```python
from build123d import *

# Parameters (mm, degrees)
SKETCH3_W           = 4
SKETCH3_H           = 0.5
BOSS_EXTRUDE1_DEPTH = 52.5
SKETCH4_R           = 0.6
CUT_EXTRUDE1_DEPTH  = 0.5
SKETCH5_R           = 0.6
CUT_EXTRUDE2_DEPTH  = 0.5
SKETCH6_R           = 0.6
CUT_EXTRUDE3_DEPTH  = 0.5
SKETCH7_R           = 0.6
CUT_EXTRUDE4_DEPTH  = 0.5
SKETCH8_R           = 0.6
CUT_EXTRUDE5_DEPTH  = 0.5
SKETCH9_R           = 0.6
CUT_EXTRUDE6_DEPTH  = 0.5
SKETCH10_R          = 0.6
CUT_EXTRUDE7_DEPTH  = 0.5
SKETCH11_R          = 0.6
CUT_EXTRUDE8_DEPTH  = 0.5
SKETCH12_R          = 0.6
CUT_EXTRUDE9_DEPTH  = 0.5
SKETCH13_R          = 0.6
CUT_EXTRUDE10_DEPTH = 0.5
SKETCH14_R          = 0.6
CUT_EXTRUDE11_DEPTH = 0.5
SKETCH15_R          = 0.6
CUT_EXTRUDE12_DEPTH = 0.5
SKETCH16_R          = 0.6
CUT_EXTRUDE13_DEPTH = 0.5
SKETCH17_R          = 0.6
CUT_EXTRUDE14_DEPTH = 0.5
SKETCH18_R          = 0.6
CUT_EXTRUDE15_DEPTH = 0.5
SKETCH19_R          = 0.6
CUT_EXTRUDE16_DEPTH = 0.5
SKETCH20_R          = 0.6
CUT_EXTRUDE17_DEPTH = 0.5
SKETCH21_R          = 0.6
CUT_EXTRUDE18_DEPTH = 0.5
SKETCH22_R          = 0.6
CUT_EXTRUDE19_DEPTH = 0.5
SKETCH23_R          = 0.6
CUT_EXTRUDE20_DEPTH = 0.3


with BuildPart() as part:
    # Sketch3 → Boss-Extrude1 (new body)
    with BuildSketch(Plane(origin=(0, 0, 0), x_dir=(1, 0, 0), z_dir=(0, 1, 0))):
        with Locations((0, 0.1)):
            Rectangle(SKETCH3_W, SKETCH3_H)
    extrude(amount=-BOSS_EXTRUDE1_DEPTH)

    # Sketch4 → Cut-Extrude1 (cut)
    with BuildSketch(Plane.XY.offset(0.15)):
        with Locations((1.25, -3.45)):
            Circle(SKETCH4_R)
    extrude(amount=-CUT_EXTRUDE1_DEPTH, mode=Mode.SUBTRACT)

    # Sketch5 → Cut-Extrude2 (cut)
    with BuildSketch(Plane.XY.offset(0.15)):
        with Locations((1.25, -5.95)):
            Circle(SKETCH5_R)
    extrude(amount=-CUT_EXTRUDE2_DEPTH, mode=Mode.SUBTRACT)

    # Sketch6 → Cut-Extrude3 (cut)
    with BuildSketch(Plane.XY.offset(0.15)):
        with Locations((1.25, -13.6)):
            Circle(SKETCH6_R)
    extrude(amount=-CUT_EXTRUDE3_DEPTH, mode=Mode.SUBTRACT)

    # Sketch7 → Cut-Extrude4 (cut)
    with BuildSketch(Plane.XY.offset(0.15)):
        with Locations((1.25, -16.1)):
            Circle(SKETCH7_R)
    extrude(amount=-CUT_EXTRUDE4_DEPTH, mode=Mode.SUBTRACT)

    # Sketch8 → Cut-Extrude5 (cut)
    with BuildSketch(Plane.XY.offset(0.15)):
        with Locations((1.25, -23.75)):
            Circle(SKETCH8_R)
    extrude(amount=-CUT_EXTRUDE5_DEPTH, mode=Mode.SUBTRACT)

    # Sketch9 → Cut-Extrude6 (cut)
    with BuildSketch(Plane.XY.offset(0.15)):
        with Locations((1.25, -26.25)):
            Circle(SKETCH9_R)
    extrude(amount=-CUT_EXTRUDE6_DEPTH, mode=Mode.SUBTRACT)

    # Sketch10 → Cut-Extrude7 (cut)
    with BuildSketch(Plane.XY.offset(0.15)):
        with Locations((1.25, -33.9)):
            Circle(SKETCH10_R)
    extrude(amount=-CUT_EXTRUDE7_DEPTH, mode=Mode.SUBTRACT)

    # Sketch11 → Cut-Extrude8 (cut)
    with BuildSketch(Plane.XY.offset(0.15)):
        with Locations((1.25, -36.4)):
            Circle(SKETCH11_R)
    extrude(amount=-CUT_EXTRUDE8_DEPTH, mode=Mode.SUBTRACT)

    # Sketch12 → Cut-Extrude9 (cut)
    with BuildSketch(Plane.XY.offset(0.15)):
        with Locations((1.25, -44.05)):
            Circle(SKETCH12_R)
    extrude(amount=-CUT_EXTRUDE9_DEPTH, mode=Mode.SUBTRACT)

    # Sketch13 → Cut-Extrude10 (cut)
    with BuildSketch(Plane.XY.offset(0.15)):
        with Locations((1.25, -46.55)):
            Circle(SKETCH13_R)
    extrude(amount=-CUT_EXTRUDE10_DEPTH, mode=Mode.SUBTRACT)

    # Sketch14 → Cut-Extrude11 (cut)
    with BuildSketch(Plane.XY.offset(0.15)):
        with Locations((-1.25, -3.45)):
            Circle(SKETCH14_R)
    extrude(amount=-CUT_EXTRUDE11_DEPTH, mode=Mode.SUBTRACT)

    # Sketch15 → Cut-Extrude12 (cut)
    with BuildSketch(Plane.XY.offset(0.15)):
        with Locations((-1.25, -5.95)):
            Circle(SKETCH15_R)
    extrude(amount=-CUT_EXTRUDE12_DEPTH, mode=Mode.SUBTRACT)

    # Sketch16 → Cut-Extrude13 (cut)
    with BuildSketch(Plane.XY.offset(0.15)):
        with Locations((-1.25, -13.6)):
            Circle(SKETCH16_R)
    extrude(amount=-CUT_EXTRUDE13_DEPTH, mode=Mode.SUBTRACT)

    # Sketch17 → Cut-Extrude14 (cut)
    with BuildSketch(Plane.XY.offset(0.15)):
        with Locations((-1.25, -16.1)):
            Circle(SKETCH17_R)
    extrude(amount=-CUT_EXTRUDE14_DEPTH, mode=Mode.SUBTRACT)

    # Sketch18 → Cut-Extrude15 (cut)
    with BuildSketch(Plane.XY.offset(0.15)):
        with Locations((-1.25, -23.75)):
            Circle(SKETCH18_R)
    extrude(amount=-CUT_EXTRUDE15_DEPTH, mode=Mode.SUBTRACT)

    # Sketch19 → Cut-Extrude16 (cut)
    with BuildSketch(Plane.XY.offset(0.15)):
        with Locations((-1.25, -26.25)):
            Circle(SKETCH19_R)
    extrude(amount=-CUT_EXTRUDE16_DEPTH, mode=Mode.SUBTRACT)

    # Sketch20 → Cut-Extrude17 (cut)
    with BuildSketch(Plane.XY.offset(0.15)):
        with Locations((-1.25, -33.9)):
            Circle(SKETCH20_R)
    extrude(amount=-CUT_EXTRUDE17_DEPTH, mode=Mode.SUBTRACT)

    # Sketch21 → Cut-Extrude18 (cut)
    with BuildSketch(Plane.XY.offset(0.15)):
        with Locations((-1.25, -36.4)):
            Circle(SKETCH21_R)
    extrude(amount=-CUT_EXTRUDE18_DEPTH, mode=Mode.SUBTRACT)

    # Sketch22 → Cut-Extrude19 (cut)
    with BuildSketch(Plane.XY.offset(0.15)):
        with Locations((-1.25, -44.05)):
            Circle(SKETCH22_R)
    extrude(amount=-CUT_EXTRUDE19_DEPTH, mode=Mode.SUBTRACT)

    # Sketch23 → Cut-Extrude20 (cut)
    with BuildSketch(Plane.XY.offset(0.15)):
        with Locations((-1.25, -46.55)):
            Circle(SKETCH23_R)
    extrude(amount=-CUT_EXTRUDE20_DEPTH, mode=Mode.SUBTRACT)


solid = part.part
```
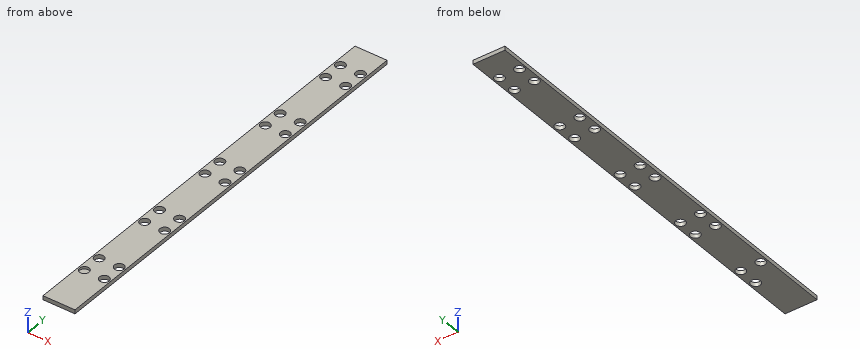
Here's how the part is built. I have some questions about the finished solid (model axes, mm). Round coordinates to 2 decimals unless told otherwise and drop trailing zeros. Write each loop counter-clockwise with the first axis right and the second up, starting at its lowest first coordinate (ties: lowest second). Pieces come first, ordered by that corner, then holes. Notation, with made-up numbers: M -29,-26.5 L -6,-26.5 A20 ccw -6,-3.5 Z; hole C -35,-30 d2. An arc over 180 degrees is marked long. Answer as CSV lines item,"result". Start each with the question number.
1. Suppose I cut it at B-B on z = -0.05. Count the separate pieces of the cut face and the enclosed holes in it, then the cut area to 3 significant figures.
2. Suppose I cut it at A-A on y = -46.55. Write out the boundary of the cut face in (x, z), then the cut area to 3 significant figures.
3. I'm going to push a flat-ended pin straight in: pin 1 Ø1.3 at (x, y) = (-1.5, -47) entering from +Z. Where does the tip first touch, or does it pass through?
4. Suppose I cut it at C-C on y = -26.25. Write out the boundary of the cut face in (x, z), then the cut area to 3 significant figures.
Check result:
1,separate pieces,"1"
1,enclosed holes,"20"
1,area,"187 mm2"
2,outline,"M -2,-0.35 L 0.65,-0.35 L 0.65,0.15 L -0.65,0.15 L -0.65,-0.15 L -1.85,-0.15 L -1.85,0.15 L -2,0.15 Z; M 1.85,-0.35 L 2,-0.35 L 2,0.15 L 1.85,0.15 Z"
2,area,"1.04 mm2"
3,pin 1,"stops at z = 0.15"
4,outline,"M -2,-0.35 L -1.85,-0.35 L -1.85,0.15 L -2,0.15 Z; M -0.65,-0.35 L 0.65,-0.35 L 0.65,0.15 L -0.65,0.15 Z; M 1.85,-0.35 L 2,-0.35 L 2,0.15 L 1.85,0.15 Z"
4,area,"0.800 mm2"
